For this review, take the finished solid that the model builds, in its own axes (mm). Round coordinates to 2 decimals unless told otherwise and drop trailing zeros. Order: outer loops, then holes, each group sorted by start corner. A loop starts at its lowest first (then second) coordinate and runs counter-clockwise, first axis right, second up. Notation, with made-up numbers: (77, 85.5) - (125, 85.5) arc R15 cw to (125, 109.5) - close; hole circle Ø10 at (60, 49.5). An arc over 180 degrees is marked (long way). One line per question, with ' | ' between items.
```python
from build123d import *

# Parameters (mm, degrees)
SKETCH1_W               = 228.6
SKETCH1_H               = 457.2
BOSS_EXTRUDE1_DEPTH     = 5.588
SKETCH2_W               = 5.588
SKETCH2_H               = 76.2
BOSS_EXTRUDE4_DEPTH     = 5.588
SKETCH3_W               = 76.2
SKETCH3_H               = 5.588
CUT_EXTRUDE1_DEPTH      = 5.588
CUT_EXTRUDE5_DEPTH      = 341.842806914
CUT_EXTRUDE5_DEPTH_BACK = 341.842806914
SKETCH4_W               = 50.8
SKETCH4_H               = 5.588


with BuildPart() as part:
    # Sketch1 → Boss-Extrude1 (new body)
    with BuildSketch(Plane.XY):
        with Locations((-78.307659574, -48.638297872)):
            Rectangle(SKETCH1_W, SKETCH1_H)
    extrude(amount=BOSS_EXTRUDE1_DEPTH)

    # Sketch2 → Boss-Extrude4 (add, through all)
    with BuildSketch(Plane.XY.offset(5.588)):
        with Locations((-195.401659574, 59.311702128)):
            Rectangle(SKETCH2_W, SKETCH2_H)
        with Locations((-195.401659574, -156.588297872)):
            Rectangle(SKETCH2_W, SKETCH2_H)
        with Locations((38.786340426, -156.588297872)):
            Rectangle(SKETCH2_W, SKETCH2_H)
        with Locations((38.786340426, 59.311702128)):
            Rectangle(SKETCH2_W, SKETCH2_H)
    extrude(amount=-BOSS_EXTRUDE4_DEPTH)

    # Sketch3 → Cut-Extrude1 (cut)
    with BuildSketch(Plane.XY.offset(5.588)):
        with Locations((-129.107659574, -274.444297872)):
            Rectangle(SKETCH3_W, SKETCH3_H)
        with Locations((-27.507659574, -274.444297872)):
            Rectangle(SKETCH3_W, SKETCH3_H)
        with Locations((-78.307659574, 177.167702128)):
            Rectangle(SKETCH3_W, SKETCH3_H)
    extrude(amount=-CUT_EXTRUDE1_DEPTH, mode=Mode.SUBTRACT)

    # Sketch4 → Cut-Extrude5 (cut, two sides: drawn at the far end of the back side and taken through both)
    with BuildSketch(Plane.XY.offset(-CUT_EXTRUDE5_DEPTH_BACK)):
        with Locations((-118.947659574, -147.444297872)):
            Rectangle(SKETCH4_W, SKETCH4_H)
        with Locations((-37.667659574, -147.444297872)):
            Rectangle(SKETCH4_W, SKETCH4_H)
    extrude(amount=CUT_EXTRUDE5_DEPTH + CUT_EXTRUDE5_DEPTH_BACK, mode=Mode.SUBTRACT)


solid = part.part
```
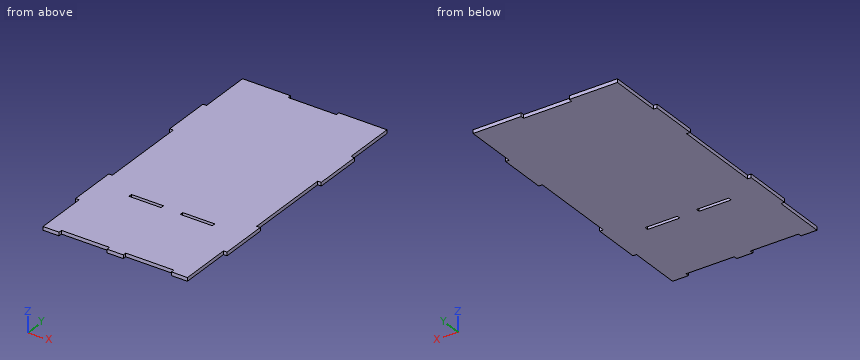
(1) We need section B-B on x = -140. State the section outline as (y, z) points.
Output values:
outline: (-271.65, 0) - (-150.24, 0) - (-150.24, 5.59) - (-271.65, 5.59) - close; (-144.65, 0) - (179.96, 0) - (179.96, 5.59) - (-144.65, 5.59) - close
(2) We need section A-A on x = -48. State the section outline as (y, z) points.
Output values:
outline: (-271.65, 0) - (-150.24, 0) - (-150.24, 5.59) - (-271.65, 5.59) - close; (-144.65, 0) - (174.37, 0) - (174.37, 5.59) - (-144.65, 5.59) - close
(3) Insertion check: pin 1 (3 mm diameter, centred on x = 38.5, z = 3, fed in from -Y); pin 2 (3 mm diameter, centred on x = -129, z = 2, fed in from -Y); pin 3 (3 mm diameter, centred on y = 177, z = 1.5, fed in from -X). Each pin has a flat end and moves straight along its axis. Give the tip position at first contact, or say it passes through.
Output values:
pin 1: y = -194.69 | pin 2: y = -271.65 | pin 3: x = -192.61
(4) We need section D-D on y = -228. State the section outline as (x, z) points.
Output values:
outline: (-192.61, 0) - (35.99, 0) - (35.99, 5.59) - (-192.61, 5.59) - close
(5) For probe 1 along Y at (x, z) = (-52, 3.6); probe 2 along Y at (x, z) = (-126, 4.6); probe 3 along Y at (x, z) = (-155, 1.8), list the stretches that pass through material, from the lowest coordinate up. Write a range as [from, to].
Output values:
probe 1: [-271.65, -150.24], [-144.65, 174.37] | probe 2: [-271.65, -150.24], [-144.65, 179.96] | probe 3: [-271.65, 179.96]
(6) We need section C-C on z = 3.55. Give the number of separate pieces and of enclosed holes in the cut face, plus the area to 3 significant figures.
Output values:
separate pieces: 1 | enclosed holes: 2 | area: 104,000 mm^2
